Verification items for the finished model (mm, model axes). Face numbers are marked on the shaded views. A direction names the side the tool comes from. Give positions to 0.01 mm unless a question says otherwise; leave off trailing zeros. Order: outer loops, then holes, each group sorted by start corner. A loop starts at its lowest first (then second) coordinate and runs counter-clockwise, first axis right, second up.
from build123d import *

# Parameters (mm, degrees)
SKETCH1_R           = 12
SKETCH1_R_2         = 7.5
BOSS_EXTRUDE1_DEPTH = 10.875
SKETCH2_R           = 0.75
BOSS_EXTRUDE2_DEPTH = 5.75
SKETCH3_R           = 7.5
BOSS_EXTRUDE3_DEPTH = 2
SKETCH4_W           = 5
SKETCH4_H           = 2
SKETCH5_R           = 1
BOSS_EXTRUDE4_DEPTH = 2
BOSS_EXTRUDE4_TAPER = 10


with BuildPart() as part:
    # Sketch1 → Boss-Extrude1 (new body)
    with BuildSketch(Plane(origin=(0, 0, 0), x_dir=(1, 0, 0), z_dir=(0, 1, 0))):
        Circle(SKETCH1_R)
        Circle(SKETCH1_R_2, mode=Mode.SUBTRACT)
    extrude(amount=BOSS_EXTRUDE1_DEPTH)

    # Sketch2 → Boss-Extrude2 (add)
    with BuildSketch(Plane(origin=(0, 10.875, 0), x_dir=(1, 0, 0), z_dir=(0, 1, 0))):
        with Locations((0, 10)):
            Circle(SKETCH2_R)
        with Locations((-8.660254038, 5)):
            Circle(SKETCH2_R)
        with Locations((-8.660254038, -5)):
            Circle(SKETCH2_R)
        with Locations((0, -10)):
            Circle(SKETCH2_R)
        with Locations((8.660254038, -5)):
            Circle(SKETCH2_R)
        with Locations((8.660254038, 5)):
            Circle(SKETCH2_R)
    extrude(amount=BOSS_EXTRUDE2_DEPTH)

    # Sketch3 → Boss-Extrude3 (add)
    with BuildSketch(Plane(origin=(0, 0, 0), x_dir=(-1, 0, 0), z_dir=(0, -1, 0))):
        Polygon((0, -9.9), (8.573651497, -4.95), (8.573651497, 4.95), (0, 9.9), (-8.573651497, 4.95), (-8.573651497, -4.95), align=None)
        Circle(SKETCH3_R, mode=Mode.SUBTRACT)
    extrude(amount=BOSS_EXTRUDE3_DEPTH)

    # Sketch4 → Revolve1 (revolve)
    with BuildSketch(Plane.XY):
        with Locations((14.5, 4.2)):
            Rectangle(SKETCH4_W, SKETCH4_H)
    revolve(axis=Axis((0, -2, 0), (0, 1, 0)))

    # Sketch5 → Boss-Extrude4 (add)
    with BuildSketch(Plane.XZ):
        with Locations((-5.25, 9.09326674)):
            Circle(SKETCH5_R)
        with Locations((5.25, 9.09326674)):
            Circle(SKETCH5_R)
        with Locations((10.5, 0)):
            Circle(SKETCH5_R)
        with Locations((5.25, -9.09326674)):
            Circle(SKETCH5_R)
        with Locations((-5.25, -9.09326674)):
            Circle(SKETCH5_R)
        with Locations((-10.5, 0)):
            Circle(SKETCH5_R)
    extrude(amount=BOSS_EXTRUDE4_DEPTH, taper=BOSS_EXTRUDE4_TAPER)


solid = part.part
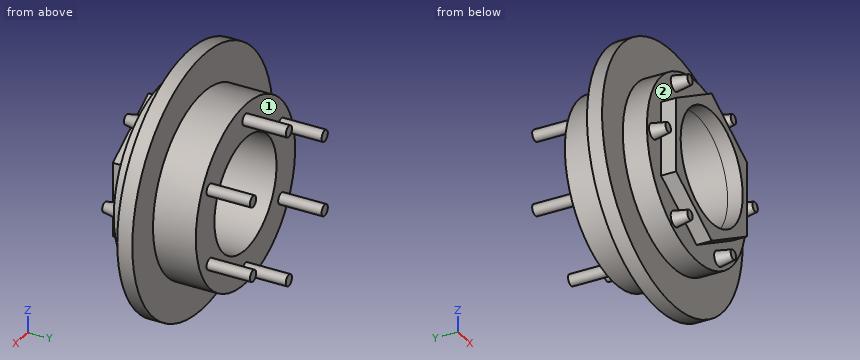
(1) Set-up check for the marked faces 1 and 2: record each of +Z, -Z, +X, -X, +Y, -Y from which the full face is reachable in a straight line by a thin tool's end or side.
Solved:
face 1: +Y
face 2: -Y
(2) Go/stop test with flat-tipped pins: pin 1 (1.5 mm diameter, centred on x = 0, y = 2, fed in from +Z); pin 2 (2 mm diameter, centred on y = 11.5, z = -1.5, fed in from -X); pin 3 (2 mm diameter, centred on y = -1.5, z = 1, fed in from +X); pin 4 (12 mm diameter, centred on x = 0, z = 0, fed in from +Y). Record where each tip stops, or that it passes through.
Solved:
pin 1: stops at z = 12
pin 2: stops at x = -11.98
pin 3: stops at x = 11.32
pin 4: passes through
(3) Section check C-C, the plane z = -7. Enter the section's corners in (x, y) (3 decimals), then the cut area to 3 significant figures.
Solved:
outline: (-15.492, 3.2) - (-9.747, 3.2) - (-9.747, 0) - (-5.023, 0) - (-5.023, -2) - (-2.693, -2) - (-2.693, 10.875) - (-9.747, 10.875) - (-9.747, 5.2) - (-15.492, 5.2) - close; (2.693, -2) - (5.023, -2) - (5.023, 0) - (9.747, 0) - (9.747, 3.2) - (15.492, 3.2) - (15.492, 5.2) - (9.747, 5.2) - (9.747, 10.875) - (2.693, 10.875) - close
area: 186 mm2
(4) Section check D-D, the plane y = 1.5. Enter the section's corners in (x, z), then the cut area to 3 significant figures.
Solved:
outline: circle Ø24 at (0, 0); hole circle Ø15 at (0, 0)
area: 276 mm2
(5) Section check A-A, the plane x = 5.25. Enter the section's corners in (y, z) (3 decimals).
Solved:
outline: (-2, -9.741) - (0, -10.093) - (0, -10.791) - (3.2, -10.791) - (3.2, -16.169) - (5.2, -16.169) - (5.2, -10.791) - (10.875, -10.791) - (10.875, -5.356) - (-2, -5.356) - (-2, -6.869) - (0, -6.869) - (0, -8.093) - (-2, -8.446) - close; (-2, 5.356) - (10.875, 5.356) - (10.875, 10.791) - (5.2, 10.791) - (5.2, 16.169) - (3.2, 16.169) - (3.2, 10.791) - (0, 10.791) - (0, 10.093) - (-2, 9.741) - (-2, 8.446) - (0, 8.093) - (0, 6.869) - (-2, 6.869) - close
(6) Scan lines: line 1 (Z direction, x = 0, y = 5.75); line 2 (Z direction, x = 0, y = -1.05); line 3 (X direction, y = 3.75, z = 0). Record each from-to range of solid material in increasing order.
Solved:
line 1: z = -12 to -7.5, 7.5 to 12
line 2: z = -9.9 to -7.5, 7.5 to 9.9
line 3: x = -17 to -7.5, 7.5 to 17
(7) Section check B-B, the plane y = 15.25. Enter the section's corners in (x, z), then the cut area to 3 significant figures.
Solved:
outline: circle Ø1.5 at (-8.66, -5); circle Ø1.5 at (-8.66, 5); circle Ø1.5 at (0, -10); circle Ø1.5 at (0, 10); circle Ø1.5 at (8.66, -5); circle Ø1.5 at (8.66, 5)
area: 10.6 mm2
